```python
from build123d import *

# Parameters (mm, degrees)
BOSS_EXTRUDE1_DEPTH = 0.2
FILLET1_R           = 0.3
FILLET2_R           = 0.03


with BuildPart() as part:
    # Sketch1 → Boss-Extrude1 (new body)
    with BuildSketch(Plane(origin=(0, 0, 0), x_dir=(1, 0, 0), z_dir=(0, 1, 0))):
        Polygon((0, 0), (0, 1.5), (0.65, 1.5), (0.65, 2), (2.75, 12), (2.75, 12.5), (3.25, 12.5), (3.25, 12.1), (4.05, 12.1), (4.05, 12.5), (4.55, 12.5), (4.55, 12), (6.65, 2), (6.65, 1.5), (7.3, 1.5), (7.3, 0), align=None)
    extrude(amount=BOSS_EXTRUDE1_DEPTH)

    # Fillet1
    fillet1_edges = [part.edges().sort_by_distance(p)[0] for p in [
        (0.65, 0.1, -1.5),
        (6.65, 0.1, -1.5),
    ]]
    fillet(fillet1_edges, radius=FILLET1_R)

    # Fillet2
    fillet2_edges = [part.edges().sort_by_distance(p)[0] for p in [
        (0, 0.1, 0),
        (0, 0.1, -1.5),
        (0.65, 0.1, -2),
        (2.75, 0.1, -12),
        (2.75, 0.1, -12.5),
        (3.25, 0.1, -12.5),
        (3.25, 0.1, -12.1),
        (4.05, 0.1, -12.1),
        (4.05, 0.1, -12.5),
        (4.55, 0.1, -12.5),
        (4.55, 0.1, -12),
        (6.65, 0.1, -2),
        (7.3, 0.1, -1.5),
        (7.3, 0.1, 0),
    ]]
    fillet(fillet2_edges, radius=FILLET2_R)


solid = part.part
```
The listing builds one solid part. Answer for the finished solid, in the listing's coordinates (mm). Give positions to 0.01 mm unless a question says otherwise; leave off trailing zeros. Order: outer loops, then holes, each group sorted by start corner. A loop starts at its lowest first (then second) coordinate and runs counter-clockwise, first axis right, second up. Notation, with made-up numbers: (-6, -20.5) - (11, -20.5) arc R13 cw to (11, -3.5) - close; hole circle Ø6 at (75.5, 88). An arc over 180 degrees is marked (long way). Use one line per item in the form item = value. Start each with the question number.
(1) Consider line 1 (X direction, y = 0.15, z = -5); line 2 (X direction, y = 0.15, z = -7.5) (3 decimals). Determine where each line is inside the solid, lowest interval first. Write a range as from..to.
(2) A cutting plane is placed at B-B, the plane z = -10. Write down the section's boundary in (x, y), then the cut area to 3 significant figures.
(3) A cutting plane is placed at C-C, the plane x = 3.5. Write down the section's boundary in (y, z), then the cut area to 3 significant figures.
Ans:
q1.line_1 = 1.28..6.02
q1.line_2 = 1.805..5.495
q2.outline = (2.33, 0) - (4.97, 0) - (4.97, 0.2) - (2.33, 0.2) - close
q2.area = 0.528 mm^2
q3.outline = (0, -12.1) - (0.2, -12.1) - (0.2, 0) - (0, 0) - close
q3.area = 2.42 mm^2
